Design review of the part built by this model. Coordinates are the model's own, in mm. A direction names the side the tool comes from. Round coordinates to 2 decimals unless told otherwise and drop trailing zeros. Loops run counter-clockwise (first coordinate to the right, second up) from the corner with the lowest first, then second, coordinate; pieces in that order, holes last. Notation, with made-up numbers: M 26.25,71.5 L 43.25,71.5 A34 ccw 43.25,108.5 Z; hole C -25.75,81 d5. An arc over 180 degrees is marked long. Use a Markdown table: item, result.
from build123d import *

# Parameters (mm, degrees)
F1_DEPTH        = 5.5
F3_DEPTH        = 4.5
F5_DEPTH        = 25.4
F5_COPIES_COUNT = 9


# Not quite as in the source:
# - a pattern or mirror of a feature is missing from the dataset's text; its kind, count and spacing are read off the source's solid


with BuildPart() as f1:
    # F0 (on Top) → F1 (new body)
    with BuildSketch(Plane.XY):
        Polygon((12.7, -4.6224219752), (12.7, 4.6224219752), (6.7575288552, 11.7043833109), (-2.3468651425, 13.3097336157), (-10.3531348575, 8.6873116405), (-13.5150577104, 0), (-10.3531348575, -8.6873116405), (-2.3468651425, -13.3097336157), (6.7575288552, -11.7043833109), align=None)
    extrude(amount=F1_DEPTH)

    # F2 (on face) → F3 (cut)
    with BuildSketch(Plane.XY.offset(5.5)):
        Polygon((3.05, -1.760918321), (3.05, 1.760918321), (0, 3.5218366421), (-3.05, 1.760918321), (-3.05, -1.760918321), (0, -3.5218366421), align=None)
    extrude(amount=-F3_DEPTH, mode=Mode.SUBTRACT)

    # F4 (on face) → F5 (cut)
    with BuildSketch(Plane.XY.offset(5.5)):
        with BuildLine():
            Line((8.4431892082, -9.6954915293), (11.014339647, -6.6313137568))
            ThreePointArc((11.014339647, -6.6313137568), (8.1966755414, -6.8778274236), (8.4431892082, -9.6954915293))
        make_face()
    f5 = extrude(amount=-F5_DEPTH, mode=Mode.SUBTRACT)

    # F5_copies: F5 ×9 about axis
    f5_copies_axis = Axis((0, 0, 0), (0, 0, 1))
    for i in range(1, F5_COPIES_COUNT):
        add(f5.rotate(f5_copies_axis, i * 360 / F5_COPIES_COUNT), mode=Mode.SUBTRACT)


solid = f1.part
1. Insertion check: pin 1 (1.5 mm diameter, centred on x = -8, z = 4, fed in from -Y); pin 2 (3 mm diameter, centred on y = 0, z = 3.5, fed in from +X); pin 3 (2 mm diameter, centred on x = -0.5, z = 2, fed in from -Y). Each pin has a flat end and moves straight along its axis. Give the tip position at first contact, or say it passes through.
Check values:
| item | result |
|---|---|
| pin 1 | stops at y = -10 |
| pin 2 | stops at x = 11.38 |
| pin 3 | stops at y = -13.16 |
2. Wall thickness on line 1 along X through (y, z) = (11, 1.75); line 2 along Y through (x, z) = (1.75, 3.55); line 3 along X through (y, z) = (-3.25, 1.35): over which ranges is each line inside the solid? List them lowest first. Write a range as from..to.
Check values:
| item | result |
|---|---|
| line 1 | x = -4.35..0.89, 3.52..7.35 |
| line 2 | y = -10.56..-2.51, 2.51..10.56 |
| line 3 | x = -10.26..-0.47, 0.47..12.7 |
3. The part is to be moulded in two halves that separate along X. For faces 1 (the face through (-3.05, 0, 3)), 2 (the face through (-3.47, 12.66, 2.71)), 3 (the face through (10.7, 0, 2.8)), say which applies: pulls with the +X half, pulls with the -X half, needs draft (parallel to the pull), parting line crosses it, or undercut.
Check values:
| item | result |
|---|---|
| face 1 | undercut |
| face 2 | pulls with the -X half |
| face 3 | pulls with the +X half |
4. Take a section at C-C on y = -4.25. Give the boundary of the cut face in (x, z), and give its area (3 significant figures).
Check values:
| item | result |
|---|---|
| outline | M -9.94,0 L 12.7,0 L 12.7,5.5 L -9.94,5.5 Z |
| area | 124 mm² |
5. Take a section at B-B on x = -6.35. Give the boundary of the cut face in (y, z), and give its area (3 significant figures).
Check values:
| item | result |
|---|---|
| outline | M -9,0 L 9,0 L 9,5.5 L -9,5.5 Z |
| area | 99.0 mm² |
6. Take a section at D-D on x = 2. Give the boundary of the cut face in (y, z), and give its area (3 significant figures).
Check values:
| item | result |
|---|---|
| outline | M -10.52,0 L 10.52,0 L 10.52,5.5 L 2.37,5.5 L 2.37,1 L -2.37,1 L -2.37,5.5 L -10.52,5.5 Z |
| area | 94.4 mm² |
7. Machinability: for faces 4 (the face through (0, 0, 1)), 5 (the face through (8.23, -6.84, 2.79)), which of the approach directions +Z, -Z, +X, -X, +Y, -Y give a long, thin tool a straight path to every point of the face, cutting with its end or side? Answer none if there is none.
Check values:
| item | result |
|---|---|
| face 4 | +Z |
| face 5 | +Z, -Z |
